Part model, mm, in its own coordinate system. A direction names the side the tool comes from. Give positions to 0.01 mm unless a question says otherwise; leave off trailing zeros. Order: outer loops, then holes, each group sorted by start corner. A loop starts at its lowest first (then second) coordinate and runs counter-clockwise, first axis right, second up. Notation, with made-up numbers: (85.5, 33.5) - (108.5, 33.5) arc R11 cw to (108.5, 47.5) - close; hole circle Ø2 at (30, 57). An arc over 180 degrees is marked (long way). Use one line per item in the form item = value. Start each with the question number.
1. Band-saw the part on D-D, the plane x = -11. List the corners of the cut face in (y, z) (1 decimal).
2. Pull direction Z, two halves, no side cores. Call faces 1 (the face through (-30.877, -0.421, -15.952)), 2 (the face through (0, 0, -7)), 3 (the face through (-30.557, 1.087, -15.736)), 4 (the face through (0, -1, -13.931)): +Z half, -Z half, draft (parallel to the pull), parting line (faces both ways), or undercut.
3. Pin check, flat tips, straight feed: P1, Ø1, axis at x = -6.5, z = -16, coming from the -Y side; P2, Ø6, axis at y = 0.5, z = -0.5, coming from the +X side; P3, Ø5, axis at y = -6.5, z = -1, coming from the -X side. Stop position of each tip, or through.
4. Band-saw the part on C-C, the plane z = -10. List the corners of the cut face in (x, y).
5. Band-saw the part on B-B, the plane y = -4. List the corners of the cut face in (x, z).
6. Band-saw the part on A-A, the plane x = -0.5. List the corners of the cut face in (y, z) (1 decimal), plus the area to 3 significant figures.
7. Tool access for faces 5 (the face through (30.557, 1.087, -15.736)), 6 (the face through (0, -2.5, -16)), 7 (the face through (0.42, 1.43, -17.33)), 8 (the face through (0, -5, 0)), 9 (the face through (0, -10.446, 1)): list every direction of +Z, -Z, +X, -X, +Y, -Y with a clear straight run to the whole face (end or side of a thin tool).
8. Drill centre lines: line 1 (Z direction, x = -13, y = -10); line 2 (Y direction, x = -17.5, z = -5.5); line 3 (X direction, y = -4.75, z = 0.5). Where is each one in solid material? Low to high.
from build123d import *

# Parameters (mm, degrees)
BOSS_EXTRUDE1_DEPTH     = 30.099
FILLET1_R               = 2
SKETCH2_W               = 1
SKETCH2_H               = 1
BOSS_EXTRUDE2_DEPTH     = 10
SKETCH3_R               = 1.5
BOSS_EXTRUDE3_DEPTH     = 1.2
CHAMFER1_SIZE           = 0.5
FILLET3_R               = 0.5
FILLET4_R               = 0.9525
CUT_EXTRUDE2_DEPTH      = 39.292428468
CUT_EXTRUDE2_DEPTH_BACK = 39.292428468


with BuildPart() as part:
    # Sketch1 → Boss-Extrude1 (new, symmetric)
    with BuildSketch(Plane(origin=(0, 0, 0), x_dir=(0, 0, -1), z_dir=(1, 0, 0))):
        Polygon((0, -10.446), (0, 0), (13.931, 0), (13.931, -2.5), (17.931, -2.5), (17.931, 2), (-1.5, 2), (-1.5, -10.446), align=None)
    extrude(amount=BOSS_EXTRUDE1_DEPTH, both=True)

    # Fillet1
    fillet1_edges = [part.edges().sort_by_distance(p)[0] for p in [
        (0, 2, -17.931),
    ]]
    fillet(fillet1_edges, radius=FILLET1_R)

    # Sketch2 → Boss-Extrude2 (add, symmetric)
    with BuildSketch(Plane(origin=(0, 0, 0), x_dir=(0, 0, -1), z_dir=(1, 0, 0))):
        with Locations((-2, -9.946)):
            Rectangle(SKETCH2_W, SKETCH2_H)
    extrude(amount=BOSS_EXTRUDE2_DEPTH, both=True)

    # Sketch3 → Boss-Extrude3 (add)
    with BuildSketch(Plane(origin=(30.099, 0, 0), x_dir=(0, 0, -1), z_dir=(1, 0, 0))):
        with Locations((15.931, -0.4)):
            Circle(SKETCH3_R)
    boss_extrude3 = extrude(amount=BOSS_EXTRUDE3_DEPTH)

    # Mirror1: Boss-Extrude3 across plane
    add(boss_extrude3.mirror(Plane(origin=(0, 0, 0), x_dir=(0, 0, 1), z_dir=(1, 0, 0))))

    # Chamfer1
    chamfer1_edges = [part.edges().sort_by_distance(p)[0] for p in [
        (-10, -9.446, 2),
        (0, -9.446, 2.5),
        (10, -9.446, 2),
    ]]
    chamfer(chamfer1_edges, length=CHAMFER1_SIZE)

    # Fillet3
    fillet3_edges = [part.edges().sort_by_distance(p)[0] for p in [
        (0, 2, 1.5),
    ]]
    fillet(fillet3_edges, radius=FILLET3_R)

    # Fillet4
    fillet4_edges = [part.edges().sort_by_distance(p)[0] for p in [
        (0, -2.5, -17.931),
        (0, -2.5, -13.931),
    ]]
    fillet(fillet4_edges, radius=FILLET4_R)

    # Sketch8 → Cut-Extrude2 (cut, two sides: drawn at the far end of the back side and taken through both)
    with BuildSketch(Plane.XY.offset(1.5).offset(-CUT_EXTRUDE2_DEPTH_BACK)):
        Polygon((30.466401846, -1.9), (31.299, 1.1), (31.299, -1.9), align=None)
        Polygon((-31.299, -1.9), (-30.466401846, -1.9), (-31.299, 1.1), align=None)
    extrude(amount=CUT_EXTRUDE2_DEPTH + CUT_EXTRUDE2_DEPTH_BACK, mode=Mode.SUBTRACT)


solid = part.part
From the geometry:
q1.outline = (-10.4, 0) - (0, 0) - (0, -13.9) - (-1.5, -13.9) arc R1 ccw to (-2.5, -14.9) - (-2.5, -17) arc R1 ccw to (-1.5, -17.9) - (0, -17.9) arc R2 ccw to (2, -15.9) - (2, 1) arc R0.5 ccw to (1.5, 1.5) - (-10.4, 1.5) - close
q2.face_1 = draft
q2.face_2 = undercut
q2.face_3 = parting line
q2.face_4 = undercut
q3.P1 = -2.5
q3.P2 = 30.1
q3.P3 = -30.1
q4.outline = (-30.1, 0) - (30.1, 0) - (30.1, 2) - (-30.1, 2) - close
q5.outline = (-30.1, 0) - (30.1, 0) - (30.1, 1.5) - (-30.1, 1.5) - close
q6.outline = (-10.4, 0) - (0, 0) - (0, -13.9) - (-1.5, -13.9) arc R1 ccw to (-2.5, -14.9) - (-2.5, -17) arc R1 ccw to (-1.5, -17.9) - (0, -17.9) arc R2 ccw to (2, -15.9) - (2, 1) arc R0.5 ccw to (1.5, 1.5) - (-9.4, 1.5) - (-9.4, 2) - (-9.9, 2.5) - (-10.4, 2.5) - close
q6.area = 64.1 mm²
q7.face_5 = +X
q7.face_6 = -Z, +X, -X, -Y
q7.face_7 = -Z, +X, -X, +Y
q7.face_8 = +X, -X, -Y
q7.face_9 = +Z, -Z, +X, -X, -Y
q8.line_1 = 0 to 1.5
q8.line_2 = 0 to 2
q8.line_3 = -30.1 to 30.1
